```python
from build123d import *

# Parameters (mm, degrees)
BOSS_EXTRU_1_DEPTH      = 7.5
CONG_1_R                = 2
ESQUISSE2_R             = 2
ENL_V_MAT_EXTRU_1_DEPTH = 3
ESQUISSE3_R             = 5.5
ENL_V_MAT_EXTRU_2_DEPTH = 51.709008317
CHANFREIN1_SIZE2        = 3.5
CHANFREIN1_SIZE         = 2.936848709
CONG_2_R                = 1.5


with BuildPart() as part:
    # Esquisse1 → Boss.-Extru.1 (new, symmetric)
    with BuildSketch(Plane(origin=(0, 0, 0), x_dir=(1, 0, 0), z_dir=(0, 1, 0))):
        with BuildLine():
            Line((3, -15), (0, -15))
            Line((0, -15), (0, 20))
            Line((0, 20), (3, 20))
            ThreePointArc((3, 20), (14.034261007, 12.998776376), (22.572863417, 22.891415916))
            Line((22.572863417, 22.891415916), (22.572863417, 37.891415916))
            ThreePointArc((22.572863417, 37.891415916), (26.572863417, 41.891415916), (30.572863417, 37.891415916))
            Line((30.572863417, 37.891415916), (30.572863417, 22.891415916))
            ThreePointArc((30.572863417, 22.891415916), (25.980595429, 10.881723069), (14.547005384, 5))
            Line((14.547005384, 5), (3, -15))
        make_face()
    extrude(amount=BOSS_EXTRU_1_DEPTH, both=True)

    # Congé1
    cong_1_edges = [part.edges().sort_by_distance(p)[0] for p in [
        (3, 0, -20),
        (14.547005384, 0, -5),
        (3, 0, 15),
    ]]
    fillet(cong_1_edges, radius=CONG_1_R)

    # Esquisse2 → Enlèv. mat.-Extru.1 (cut)
    with BuildSketch(Plane.ZY):
        Circle(ESQUISSE2_R)
    extrude(amount=-ENL_V_MAT_EXTRU_1_DEPTH, mode=Mode.SUBTRACT)

    # Esquisse3 → Enlèv. mat.-Extru.2 (cut, through all)
    with BuildSketch(Plane.ZY.offset(-3)):
        Circle(ESQUISSE3_R)
    extrude(amount=-ENL_V_MAT_EXTRU_2_DEPTH, mode=Mode.SUBTRACT)

    # Chanfrein1
    chanfrein1_edges = [part.edges().sort_by_distance(p)[0] for p in [
        (3, 0, -5.5),
    ]]
    chanfrein1_side = [part.faces().sort_by_distance(p)[0] for p in [
        (3.058736974, 0, -5.5),
    ]]
    chamfer(chanfrein1_edges, length=CHANFREIN1_SIZE - 0.0001, length2=CHANFREIN1_SIZE2 - 0.0001, reference=chanfrein1_side[0])  # a hair under: the kernel refuses the full size

    # Congé2
    cong_2_edges = [part.edges().sort_by_distance(p)[0] for p in [
        (30.572863417, -7.5, -30.391415916),
        (0.922649731, -7.5, 15),
        (30.572863417, 7.5, -30.391415916),
        (26.572863417, 7.5, -41.891415916),
        (22.572863417, 7.5, -30.391415916),
        (14.656699474, 7.5, -13.110944185),
        (0.807516434, -7.5, -20),
        (0.807516434, 7.5, -20),
        (26.286115703, -7.5, -11.231797066),
        (8.81730911, -7.5, 4.924125057),
        (2.845299462, -7.5, 14.732050808),
        (2.703501524, -7.5, -19.677866498),
        (8.81730911, 7.5, 4.924125057),
        (26.286115703, 7.5, -11.231797066),
        (2.845299462, 7.5, 14.732050808),
        (2.703501524, 7.5, -19.677866498),
        (14.652846189, -7.5, -4.797480755),
        (14.652846189, 7.5, -4.797480755),
        (0.922649731, 7.5, 15),
        (14.656699474, -7.5, -13.110944185),
        (22.572863417, -7.5, -30.391415916),
        (26.572863417, -7.5, -41.891415916),
    ]]
    fillet(cong_2_edges, radius=CONG_2_R)


solid = part.part
```
Can you work these out from the model? Positions are in its coordinate system, mm. A direction names the side the tool comes from. Give positions to 0.01 mm unless a question says otherwise; leave off trailing zeros. Loops run counter-clockwise (first coordinate to the right, second up) from the corner with the lowest first, then second, coordinate; pieces in that order, holes last. Notation, with made-up numbers: M 75.25,30.25 L 91.25,30.25 A25 cw 91.25,51.25 Z; hole C 53.5,19 d4. An arc over 180 degrees is marked long. One line per item, written item: value.
(1) I need wall thicknesses on line 1 (Y direction, x = 1, z = 0); line 2 (Y direction, x = 10, z = 0); line 3 (X direction, y = 2.75, z = -29). Which ranges of each line are inside material? Lowest first, please.
Returned:
line 1: -7.5 to -2, 2 to 7.5
line 2: -7.5 to -5.5, 5.5 to 7.5
line 3: 22.57 to 30.57
(2) Will these pins go through, and if not, where does the flat tip stop? pin 1 (5 mm diameter, centred on x = 15, y = 3.5, fed in from +Z); pin 2 (5 mm diameter, centred on y = 4.5, z = -8.5, fed in from +X); pin 3 (0.5 mm diameter, centred on x = 1, y = 0.5, fed in from -Z).
Returned:
pin 1: z = -2.31
pin 2: x = 26.09
pin 3: z = -20
(3) We'd pull the mould along Z, two halves only. Please class faces 5 (the face through (0, 0.1, -2.3)), 6 (the face through (0.91, -7.07, 14.55)), 7 (the face through (1, -2, 0)), 8 (the face through (8.99, 0.242, -5.495)): released by +Z, released by -Z, zero draft, split by the parting line, or undercut.
Returned:
face 5: zero draft
face 6: released by +Z
face 7: undercut
face 8: undercut
(4) Which directions (+Z, -Z, +X, -X, +Y, -Y) give clear straight access to the entire face, cutting with the end or side of a thin tool? Please do faces 1 (the face through (1, 0, -20)), 2 (the face through (2.717, -0.084, -19.669)), 3 (the face through (23.02, -7.07, -30.5)), 4 (the face through (23.02, 7.07, -30.5)).
Returned:
face 1: -Z, -X, +Y, -Y
face 2: -Z, +Y, -Y
face 3: -Z, -X, -Y
face 4: -Z, -X, +Y
(5) Suppose I cut it at A-A on z = -27.5. List the corners of the cut face in (x, y) for me, plus the area to 3 significant figures.
Returned:
outline: M 22.57,-6 A1.5 ccw 24.07,-7.5 L 29.07,-7.5 A1.5 ccw 30.57,-6 L 30.57,6 A1.5 ccw 29.07,7.5 L 24.07,7.5 A1.5 ccw 22.57,6 Z
area: 118 mm^2
